Read the model definition and answer for the solid it produces. Units are mm, in the model's axes. Face numbers are marked on the shaded views. A direction names the side the tool comes from. Round coordinates to 2 decimals unless told otherwise and drop trailing zeros. Use CSV: the item, a comma, the result in double quotes. Start each with the question number.
1. Consider line 1 along X through (y, z) = (15, 24.5); line 2 along X through (y, z) = (34, 49); line 3 along X through (y, z) = (37, 49). Determine where each line is inside the solid, lowest interval first.
2. A tool of negligible diameter and unlimited length cuts with its end or side. For the marked faces 1, 2, 3, 4 and 5, from which of +Z, -Z, +X, -X, +Y, -Y can it reach the whole face along a straight path? Write none if from no direction.
3. Given pin 1 Ø1 at (x, y) = (29, 11) entering from +Z; pin 2 Ø6.5 at (x, z) = (9.5, 49) entering from -Y; pin 3 Ø1 at (y, z) = (31, 8) entering from +X (3 decimals); pin 4 Ø4.5 at (x, y) = (15, 15) entering from -Z, each flat-ended and moving along its own axis, determine where each tip first touches the part or whether it passes through.
4. Find section A-A (x = 15). State how many separate pieces and enclosed holes the cut face has, and give its area (3 significant figures).
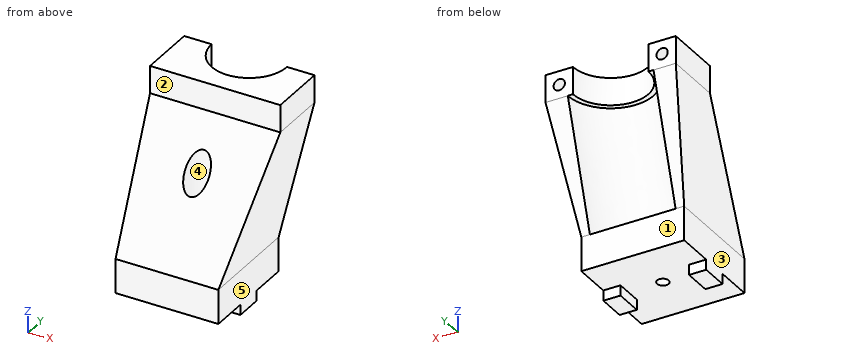
from build123d import *

# Parameters (mm, degrees)
SKETCH_1_W          = 30
SKETCH_1_H          = 30
EXTRUDE_1_DEPTH     = 10
EXTRUDE_3_DEPTH     = 8
SKETCH_11_R         = 3.5
CUT_EXTRUDE_2_DEPTH = 69.45436447
SKETCH_12_W         = 5
SKETCH_12_H         = 8.1
EXTRUDE_4_DEPTH     = 3


with BuildPart() as part:
    # Sketch 1 → Extrude 1 (new body)
    with BuildSketch(Plane.XY):
        with Locations((15, 15)):
            Rectangle(SKETCH_1_W, SKETCH_1_H)
    extrude(amount=EXTRUDE_1_DEPTH)

    # Other 1: read off the stored shape, not the designer's step
    # Other 1 outline → Other 1 (revolve, cut)
    with BuildSketch(Plane(origin=(15, 15, 0), x_dir=(1, 0, 0), z_dir=(0, -1, 0))):
        Polygon((3.15, 10), (0, 10), (0, 0), (1.7, 0), (1.7, 8.55), align=None)
    revolve(axis=Axis((15, 15, 0), (0, 0, 1)), mode=Mode.SUBTRACT)



with BuildPart() as body_2:
    # Sketch 2 → Extrude 3 (new body)
    with BuildSketch(Plane.XY.offset(45)):
        with BuildLine():
            Line((-4, 41), (4, 41))
            ThreePointArc((4, 41), (15, 30), (26, 41))
            Line((26, 41), (34, 41))
            Line((34, 41), (34, 24))
            Line((34, 24), (-4, 24))
            Line((-4, 24), (-4, 41))
        make_face()
    extrude(amount=EXTRUDE_3_DEPTH)


with BuildPart() as part_1:
    add(part.part)

    add(body_2.part)  # Loft 2 merges body 2
    # Sketch 3 → Loft 2 section 0
    with BuildSketch(Plane(origin=(0, 0, 45), x_dir=(-1, 0, 0), z_dir=(0, 0, -1))):
        with BuildLine():
            Line((-34, 41), (-27.5, 41))
            ThreePointArc((-27.5, 41), (-15, 28.5), (-2.5, 41))
            Line((-2.5, 41), (4, 41))
            Line((4, 41), (4, 24))
            Line((4, 24), (-34, 24))
            Line((-34, 24), (-34, 41))
        make_face()
    # Sketch 5 → Loft 2 section 1
    with BuildSketch(Plane.XY.offset(10)):
        with BuildLine():
            Line((27.5, 30), (30, 30))
            Line((30, 30), (30, 0))
            Line((30, 0), (0, 0))
            Line((0, 0), (0, 30))
            Line((0, 30), (2.5, 30))
            ThreePointArc((2.5, 30), (15, 17.5), (27.5, 30))
        make_face()
    loft()

    # Sketch 11 → Cut-Extrude 2 (cut, through all)
    with BuildSketch(Plane(origin=(0, 0, 10), x_dir=(-1, 0, 0), z_dir=(0, 0, -1))):
        with Locations(Location((-15, 15, 0), (0, 0, 50.487533502))):
            Circle(SKETCH_11_R)
    extrude(amount=-CUT_EXTRUDE_2_DEPTH, mode=Mode.SUBTRACT)

    # Sketch 12 → Extrude 4 (add)
    with BuildSketch(Plane(origin=(0, 0, 0), x_dir=(-1, 0, 0), z_dir=(0, 0, -1))):
        with Locations((-27.5, 15)):
            Rectangle(SKETCH_12_W, SKETCH_12_H)
        with Locations((-2.5, 15)):
            Rectangle(SKETCH_12_W, SKETCH_12_H)
    extrude(amount=EXTRUDE_4_DEPTH)

    # Other 4: read off the stored shape, not the designer's step
    # Other 4 outline → Other 4 (revolve, cut)
    with BuildSketch(Plane(origin=(30, 0, 49), x_dir=(1, 0, 0), z_dir=(0, 0, 1))):
        Polygon((0, 30.008579979), (1.65, 31), (1.65, 41), (0, 41), align=None)
    revolve(axis=Axis((30, 0, 49), (0, 1, 0)), mode=Mode.SUBTRACT)

    # Other 4 2 outline → Other 4 2 (revolve, cut)
    with BuildSketch(Plane.XY.offset(49)):
        Polygon((0, 30.008579979), (1.65, 31), (1.65, 41), (0, 41), align=None)
    revolve(axis=Axis((0, 0, 49), (0, 1, 0)), mode=Mode.SUBTRACT)


solid = part_1.part
Filled sheet:
1,line 1,"x = -1.66 to 11.5, 18.5 to 31.66"
1,line 2,"x = -4 to -1.65, 1.65 to 6.51, 23.49 to 28.35, 31.65 to 34"
1,line 3,"x = -4 to -1.65, 1.65 to 4.75, 25.25 to 28.35, 31.65 to 34"
2,face 1,"-Z, +X, -X, +Y"
2,face 2,"+Z, +X, -X, -Y"
2,face 3,"-Z, -X, +Y, -Y"
2,face 4,"+Z"
2,face 5,"-Z, +X, +Y, -Y"
3,pin 1,"stops at z = 26.77"
3,pin 2,"stops at y = 24"
3,pin 3,"passes through"
3,pin 4,"stops at z = 0"
4,separate pieces,"3"
4,enclosed holes,"0"
4,area,"545 mm²"
